Here's how the part is built. I have some questions about the finished solid (model axes, mm). Face numbers are marked on the shaded views. A direction names the side the tool comes from. Round coordinates to 2 decimals unless told otherwise and drop trailing zeros. Order: outer loops, then holes, each group sorted by start corner. A loop starts at its lowest first (then second) coordinate and runs counter-clockwise, first axis right, second up.
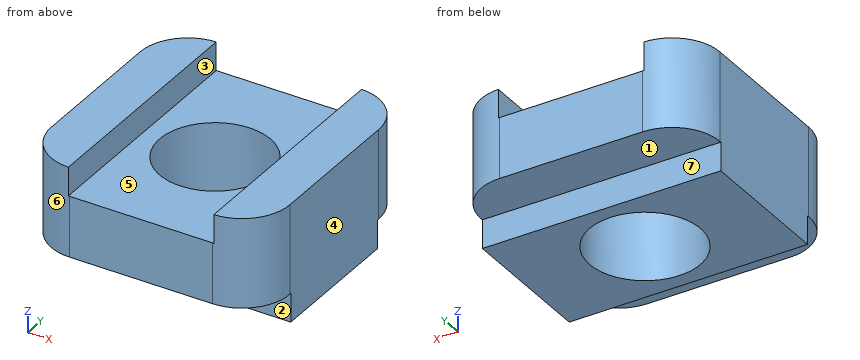
Autodesk Inventor part; units mm, degrees
ref_plane "YZ Plane" through (0, 0, 0) normal (1, 0, 0) x (0, 1, 0)
ref_plane "XZ Plane" through (0, 0, 0) normal (0, 1, 0) x (-1, 0, 0)
ref_plane "XY Plane" through (0, 0, 0) normal (0, 0, 1) x (1, 0, 0)
sketch "Sketch1" plane through (0, 0, 0) normal (1, 0, 0) x (0, 1, 0)
  line L0 (-20, 7.5) -> (20, 7.5)
  line L1 (20, 7.5) -> (20, -7.5)
  line L2 (20, -7.5) -> (11.75, -7.5)
  line L3 (11.75, -7.5) -> (11.75, -12.3)
  line L4 (11.75, -12.3) -> (-11.75, -12.3)
  line L5 (-11.75, -12.3) -> (-11.75, -7.5)
  line L6 (-11.75, -7.5) -> (-20, -7.5)
  line L7 (-20, -7.5) -> (-20, 7.5)
  point P0 (0, 0)
  point P1 (0, 7.5)
  point P2 (20, 0)
  point P3 (0, -12.3)
  dimension "d0" = 15
  dimension "d1" = 40
  dimension "d2" = 4.8
  dimension "d3" = 23.5
extrude "Extrusion1" add sketch "Sketch1" along normal mid plane 40
sketch "Sketch2" plane through (-20, 20, 7.5) normal (0, 1, 0) x (1, 0, 0)
  line L0 (32.2, 0) -> (7.8, 0)
  line L1 (7.8, 0) -> (7.8, 4.8)
  line L2 (7.8, 4.8) -> (32.2, 4.8)
  line L3 (32.2, 4.8) -> (32.2, 0)
  point P0 (20, 7.5)
  point P1 (40, 0)
  point P2 (20, 4.8)
  dimension "d6" = 24.4
  dimension "d7" = 4.8
extrude "Extrusion2" cut sketch "Sketch2" against normal up to next
fillet "Fillet1" radius 8 4 edges at (20, 20, 0) (-20, 20, 0) (-20, -20, 0) (20, -20, 0)
sketch "Sketch3" plane through (-12, 20, 2.7) normal (0, 0, 1) x (1, 0, 0)
  circle A0 centre (12, -20) radius 9.3
  dimension "d11" = 18.6
extrude "Extrusion3" cut sketch "Sketch3" against normal up to next
properties part number "OldhamCouplerMiddle"
1. If we section it at C-C, the plane y = -2: Write out the boundary of the cut face in (x, z).
Evaluation:
outline: (-20, -12.3) - (-9.08, -12.3) - (-9.08, 2.7) - (-12.2, 2.7) - (-12.2, 7.5) - (-20, 7.5) - close; (9.08, -12.3) - (20, -12.3) - (20, 7.5) - (12.2, 7.5) - (12.2, 2.7) - (9.08, 2.7) - close
2. On a 3-axis mill with a long thin cutter (end or side, diameter ignored), from which of +Z, -Z, +X, -X, +Y, -Y can I reach the whole of each face in a straight line? I mean the marked faces 1, 2, 3 and 4. Say none if no direction works.
Evaluation:
face 1: -Z, +X, -X, +Y
face 2: -Z, +X, -X, -Y
face 3: +Z, +Y, -Y
face 4: +Z, -Z, +X, +Y, -Y
3. I'm going to push flat-ended pins straight in: P1, Ø7.5, axis at x = -6, y = 5, coming from the +Z side; P2, Ø2.5, axis at x = -0.5, z = -10.5, coming from the +Y side; P3, Ø4, axis at x = -7.5, y = 16.5, coming from the -Z side. Where does each tip first touch, or does it pass through?
Evaluation:
P1: stops at z = 2.7
P2: stops at y = 11.75
P3: stops at z = -7.5
4. If we mould it in two halves opening along X, with no side actions, what happens to the marked faces 5, 6 and 7? For each: released by +X, released by -X, zero draft, split by the parting line, or undercut.
Evaluation:
face 5: undercut
face 6: released by -X
face 7: zero draft
5. I need wall thicknesses on probe 1 along X at (y, z) = (-7.5, 5.25); probe 2 along Z at (x, y) = (15, 14); probe 3 along Z at (x, y) = (4, 8.5). Which ranges of each line are inside material? Lowest first, please.
Evaluation:
probe 1: x = -20 to -12.2, 12.2 to 20
probe 2: z = -7.5 to 7.5
probe 3: z = -12.3 to 2.7
6. If we section it at D-D, the plane x = 10: Write out the boundary of the cut face in (y, z), and give its area (3 significant figures).
Evaluation:
outline: (-20, -7.5) - (-11.75, -7.5) - (-11.75, -12.3) - (11.75, -12.3) - (11.75, -7.5) - (20, -7.5) - (20, 2.7) - (-20, 2.7) - close
area: 521 mm2
7. If we section it at A-A, the plane x = 0: Write out the boundary of the cut face in (y, z).
Evaluation:
outline: (-20, -7.5) - (-11.75, -7.5) - (-11.75, -12.3) - (-9.3, -12.3) - (-9.3, 2.7) - (-20, 2.7) - close; (9.3, -12.3) - (11.75, -12.3) - (11.75, -7.5) - (20, -7.5) - (20, 2.7) - (9.3, 2.7) - close
8. If we section it at B-B, the plane z = -3: Write out the boundary of the cut face in (x, y), and give its area (3 significant figures).
Evaluation:
outline: (-20, -12) arc R8 ccw to (-12, -20) - (12, -20) arc R8 ccw to (20, -12) - (20, 12) arc R8 ccw to (12, 20) - (-12, 20) arc R8 ccw to (-20, 12) - close; hole circle Ø18.6 at (0, 0)
area: 1,270 mm2
